Read the model definition and answer for the solid it produces. Units are mm, in the model's axes. Face numbers are marked on the shaded views. A direction names the side the tool comes from. Coordinates: 2 decimals unless noted, no trailing zeros. Loops run counter-clockwise (first coordinate to the right, second up) from the corner with the lowest first, then second, coordinate; pieces in that order, holes last.
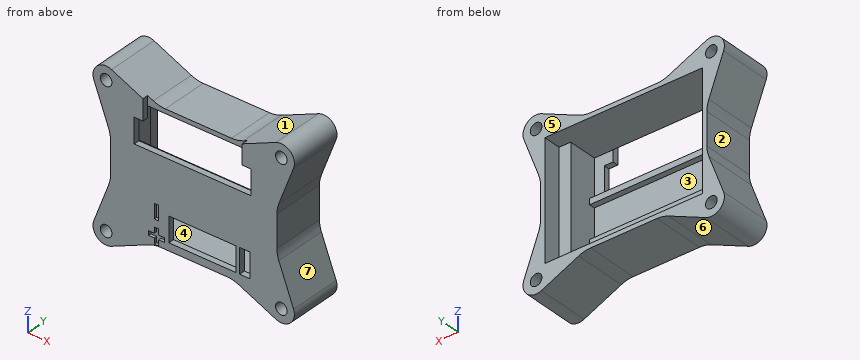
from build123d import *

# Parameters (mm, degrees)
SKETCH1_R           = 2
SKETCH1_W           = 57
SKETCH1_H           = 43
SKETCH1_W_2         = 54
SKETCH1_H_2         = 40
BOSS_EXTRUDE1_DEPTH = 18
SKETCH2_W           = 2.5
SKETCH2_H           = 40
SKETCH2_W_2         = 4
BOSS_EXTRUDE2_DEPTH = 12
SKETCH3_W           = 54
SKETCH3_H           = 40
SKETCH3_W_2         = 40
SKETCH3_H_2         = 8.5
SKETCH3_W_3         = 23
SKETCH3_W_4         = 3.5
BOSS_EXTRUDE3_DEPTH = 2
SKETCH4_W           = 1.5
SKETCH4_H           = 5
CUT_EXTRUDE1_DEPTH  = 1
BOSS_EXTRUDE4_REACH = 59.5
SKETCH5_W           = 2
SKETCH5_H           = 2
FILLET1_R           = 10
CUT_EXTRUDE2_START  = -5.35
SKETCH6_W           = 34
SKETCH6_H           = 2
CUT_EXTRUDE2_DEPTH  = 7.103529


with BuildPart() as part:
    # Sketch1 → Boss-Extrude1 (new body)
    with BuildSketch(Plane(origin=(0, 0, 0), x_dir=(1, 0, 0), z_dir=(0, 1, 0))):
        with BuildLine():
            Line((-28.5, 7.357542402), (-28.5, 21.5))
            Line((-28.5, 21.5), (-13.47815401, 21.5))
            Line((-13.47815401, 21.5), (-28.153404403, 28.103667226))
            ThreePointArc((-28.153404403, 28.103667226), (-33.084632617, 27.276437336), (-34.207471192, 22.404009346))
            Line((-34.207471192, 22.404009346), (-28.5, 7.357542402))
        make_face()
        with Locations((-30, 24)):
            Circle(SKETCH1_R, mode=Mode.SUBTRACT)
        with BuildLine():
            Line((-28.5, -21.5), (-28.5, -7.357542402))
            Line((-28.5, -7.357542402), (-34.207471192, -22.404009346))
            ThreePointArc((-34.207471192, -22.404009346), (-33.084632617, -27.276437336), (-28.153404403, -28.103667226))
            Line((-28.153404403, -28.103667226), (-13.47815401, -21.5))
            Line((-13.47815401, -21.5), (-28.5, -21.5))
        make_face()
        with Locations((-30, -24)):
            Circle(SKETCH1_R, mode=Mode.SUBTRACT)
        Rectangle(SKETCH1_W, SKETCH1_H)
        Rectangle(SKETCH1_W_2, SKETCH1_H_2, mode=Mode.SUBTRACT)
        with BuildLine():
            Line((34.207471192, -22.404009346), (28.5, -7.357542402))
            Line((28.5, -7.357542402), (28.5, -21.5))
            Line((28.5, -21.5), (13.47815401, -21.5))
            Line((13.47815401, -21.5), (28.153404403, -28.103667226))
            ThreePointArc((28.153404403, -28.103667226), (33.084632617, -27.276437336), (34.207471192, -22.404009346))
        make_face()
        with Locations((30, -24)):
            Circle(SKETCH1_R, mode=Mode.SUBTRACT)
        with BuildLine():
            Line((28.153404403, 28.103667226), (13.47815401, 21.5))
            Line((13.47815401, 21.5), (28.5, 21.5))
            Line((28.5, 21.5), (28.5, 7.357542402))
            Line((28.5, 7.357542402), (34.207471192, 22.404009346))
            ThreePointArc((34.207471192, 22.404009346), (33.084632617, 27.276437336), (28.153404403, 28.103667226))
        make_face()
        with Locations((30, 24)):
            Circle(SKETCH1_R, mode=Mode.SUBTRACT)
    extrude(amount=BOSS_EXTRUDE1_DEPTH)

    # Sketch2 → Boss-Extrude2 (add)
    with BuildSketch(Plane(origin=(0, 0, 0), x_dir=(1, 0, 0), z_dir=(0, 1, 0))):
        with Locations((-25.75, 0)):
            Rectangle(SKETCH2_W, SKETCH2_H)
        with Locations((25, 0)):
            Rectangle(SKETCH2_W_2, SKETCH2_H)
    extrude(amount=BOSS_EXTRUDE2_DEPTH)

    # Sketch3 → Boss-Extrude3 (add)
    with BuildSketch(Plane(origin=(0, 0, 0), x_dir=(1, 0, 0), z_dir=(0, 1, 0))):
        Rectangle(SKETCH3_W, SKETCH3_H)
        with Locations((-0.375, -11.9)):
            Rectangle(SKETCH3_W_2, SKETCH3_H_2, mode=Mode.SUBTRACT)
        with Locations((3, 14.65)):
            Rectangle(SKETCH3_W_3, SKETCH3_H_2, mode=Mode.SUBTRACT)
        with Locations((17.5, 14.65)):
            Rectangle(SKETCH3_W_4, SKETCH3_H_2, mode=Mode.SUBTRACT)
    extrude(amount=BOSS_EXTRUDE3_DEPTH)

    # Sketch4 → Cut-Extrude1 (cut)
    with BuildSketch(Plane.XZ):
        Polygon((-10, -17.9), (-10, -19.4), (-12, -19.4), (-12, -21.4), (-13.5, -21.4), (-13.5, -19.4), (-15.5, -19.4), (-15.5, -17.9), (-13.5, -17.9), (-13.5, -15.9), (-12, -15.9), (-12, -17.9), align=None)
        with Locations((-12.75, -10.9)):
            Rectangle(SKETCH4_W, SKETCH4_H)
    extrude(amount=-CUT_EXTRUDE1_DEPTH, mode=Mode.SUBTRACT)

    # Sketch5 → Boss-Extrude4 (add, up to next)
    with BuildSketch(Plane.ZY.offset(-23), mode=Mode.PRIVATE) as boss_extrude4_sk1:
        with Locations((5.15, 3)):
            Rectangle(SKETCH5_W, SKETCH5_H)
    boss_extrude4_tool1 = extrude(boss_extrude4_sk1.sketch, amount=BOSS_EXTRUDE4_REACH, mode=Mode.PRIVATE) - part.part
    add(boss_extrude4_tool1.solids().sort_by_distance((23, 3, 5.15))[0])
    # Sketch5 → Boss-Extrude4 (add, up to next)
    with BuildSketch(Plane.ZY.offset(-23), mode=Mode.PRIVATE) as boss_extrude4_sk2:
        with Locations((-7.9, 3)):
            Rectangle(SKETCH5_W, SKETCH5_H)
    boss_extrude4_tool2 = extrude(boss_extrude4_sk2.sketch, amount=BOSS_EXTRUDE4_REACH, mode=Mode.PRIVATE) - part.part
    add(boss_extrude4_tool2.solids().sort_by_distance((23, 3, -7.9))[0])

    # Fillet1
    fillet1_edges = [part.edges().sort_by_distance(p)[0] for p in [
        (28.5, 9, 7.357542402),
        (13.47815401, 9, 21.5),
        (-13.47815401, 9, 21.5),
        (-28.5, 9, 7.357542402),
        (-28.5, 9, -7.357542402),
        (-13.47815401, 9, -21.5),
        (13.47815401, 9, -21.5),
        (28.5, 9, -7.357542402),
    ]]
    fillet(fillet1_edges, radius=FILLET1_R)

    # Sketch6 → Cut-Extrude2 (cut)
    with BuildSketch(Plane.XY.offset(21.5).offset(CUT_EXTRUDE2_START)):
        with Locations((-0.375, 1)):
            Rectangle(SKETCH6_W, SKETCH6_H)
    extrude(amount=CUT_EXTRUDE2_DEPTH, mode=Mode.SUBTRACT)


solid = part.part
Item 1: A cutting plane is placed at B-B on y = 7.25. Give the number of separate pieces and of enclosed holes in the cut face, then the cut area to 3 significant figures.
Numbers:
separate pieces: 1
enclosed holes: 5
area: 1,010 mm2
Item 2: Find the intervals of material crossed by line 1 along Z through (x, y) = (-0.5, 9.75); line 2 along X through (y, z) = (5.25, -24); line 3 along X through (y, z) = (16.25, -23.5), in increasing order.
Numbers:
line 1: z = -21.5 to -20, 20 to 21.5
line 2: x = -34.5 to -32, -28 to -19.03, 19.03 to 28, 32 to 34.5
line 3: x = -34.47 to -31.94, -28.06 to -17.92, 17.92 to 28.06, 31.94 to 34.47
Item 3: Determine the mould class of the marked faces 4, 5, 6 and 7 for opening direction X: released by +X, released by -X, zero draft, split by the parting line, or undercut.
Numbers:
face 4: undercut
face 5: zero draft
face 6: undercut
face 7: released by +X
Item 4: Given pin 1 (3 mm diameter, centred on y = 2.5, z = -10.5, fed in from +X); pin 2 (3 mm diameter, centred on x = -10, z = -18, fed in from +Y); pin 3 (10 mm diameter, centred on y = 3, z = 13, fed in from -X), each flat-ended and moving along its own axis, determine where each tip first touches the part or whether it passes through.
Numbers:
pin 1: stops at x = 30.26
pin 2: stops at y = 2
pin 3: stops at x = -32.54
Item 5: Which of the six approach directions +Z, -Z, +X, -X, +Y, -Y give full straight-line access (tool end or side, diameter ignored) to the marked faces 1, 2 and 3?
Numbers:
face 1: +Z, +Y, -Y
face 2: -X, +Y, -Y
face 3: +Y
Item 6: A cutting plane is placed at A-A on x = 4. Determine the outline of the cut face in (y, z).
Numbers:
outline: (0, -21.5) - (18, -21.5) - (18, -20) - (2, -20) - (2, -18.9) - (0, -18.9) - close; (0, -10.4) - (2, -10.4) - (2, -8.9) - (4, -8.9) - (4, -6.9) - (2, -6.9) - (2, 4.15) - (4, 4.15) - (4, 6.15) - (2, 6.15) - (2, 7.65) - (0, 7.65) - close; (2, 20) - (18, 20) - (18, 21.5) - (2, 21.5) - close
Item 7: A cutting plane is placed at C-C on z = 17.5. Determine the outline of the cut face in (x, y) (3 decimals).
Numbers:
outline: (-32.347, 0) - (-17.375, 0) - (-17.375, 2) - (-24.5, 2) - (-24.5, 12) - (-27, 12) - (-27, 18) - (-32.347, 18) - close; (16.625, 0) - (32.347, 0) - (32.347, 18) - (27, 18) - (27, 12) - (23, 12) - (23, 2) - (16.625, 2) - close
Item 8: A cutting plane is placed at D-D on z = 24. Determine the outline of the cut face in (x, y).
Numbers:
outline: (-34.5, 0) - (-32, 0) - (-32, 18) - (-34.5, 18) - close; (-28, 0) - (-19.03, 0) - (-19.03, 18) - (-28, 18) - close; (19.03, 0) - (28, 0) - (28, 18) - (19.03, 18) - close; (32, 0) - (34.5, 0) - (34.5, 18) - (32, 18) - close
